Source: CAD feature listing. Evaluate the final solid. Frame: model axes, mm. A direction names the side the tool comes from. Give positions to 0.01 mm unless a question says otherwise; leave off trailing zeros. Order: outer loops, then holes, each group sorted by start corner. A loop starts at its lowest first (then second) coordinate and runs counter-clockwise, first axis right, second up. Notation, with made-up numbers: (13, 5.5) - (51, 5.5) arc R8 ccw to (51, 19.5) - close; hole circle Ø8 at (6, 35). An arc over 180 degrees is marked (long way). Use CSV: the item, a comma, the result in double quotes.
```python
from build123d import *

# Parameters (mm, degrees)
SKETCH1_R           = 1.5
BOSS_EXTRUDE1_DEPTH = 1.75
BOSS_EXTRUDE2_DEPTH = 3
BOSS_EXTRUDE3_DEPTH = 0.5
CUT_EXTRUDE1_REACH  = 5.5
SKETCH4_R           = 0.311736168


with BuildPart() as part:
    # Sketch1 → Boss-Extrude1 (new body)
    with BuildSketch(Plane(origin=(0, 0, 0), x_dir=(1, 0, 0), z_dir=(0, 1, 0))):
        with BuildLine():
            Line((16, -18), (-16, -18))
            ThreePointArc((-16, -18), (-17.414213562, -17.414213562), (-18, -16))
            Line((-18, -16), (-18, 16))
            ThreePointArc((-18, 16), (-17.414213562, 17.414213562), (-16, 18))
            Line((-16, 18), (16, 18))
            ThreePointArc((16, 18), (17.414213562, 17.414213562), (18, 16))
            Line((18, 16), (18, -16))
            ThreePointArc((18, -16), (17.414213562, -17.414213562), (16, -18))
        make_face()
        with Locations((15.25, 15.25)):
            Circle(SKETCH1_R, mode=Mode.SUBTRACT)
        with Locations((-15.25, 15.25)):
            Circle(SKETCH1_R, mode=Mode.SUBTRACT)
        with Locations((15.25, -15.25)):
            Circle(SKETCH1_R, mode=Mode.SUBTRACT)
        with Locations((-15.25, -15.25)):
            Circle(SKETCH1_R, mode=Mode.SUBTRACT)
    extrude(amount=BOSS_EXTRUDE1_DEPTH)

    # Sketch2 → Boss-Extrude2 (add)
    with BuildSketch(Plane.XY.offset(18)):
        with BuildLine():
            Line((4.625773415, 1.75), (8.625773415, 1.75))
            Line((8.625773415, 1.75), (8.625773415, 3.25))
            ThreePointArc((8.625773415, 3.25), (8.596484093, 3.320710678), (8.525773415, 3.35))
            Line((8.525773415, 3.35), (8.325773415, 3.35))
            ThreePointArc((8.325773415, 3.35), (8.255062737, 3.379289322), (8.225773415, 3.45))
            Line((8.225773415, 3.45), (8.225773415, 3.65))
            ThreePointArc((8.225773415, 3.65), (8.196484093, 3.720710678), (8.125773415, 3.75))
            Line((8.125773415, 3.75), (5.125773415, 3.75))
            ThreePointArc((5.125773415, 3.75), (5.055062737, 3.720710678), (5.025773415, 3.65))
            Line((5.025773415, 3.65), (5.025773415, 3.45))
            ThreePointArc((5.025773415, 3.45), (4.996484093, 3.379289322), (4.925773415, 3.35))
            Line((4.925773415, 3.35), (4.725773415, 3.35))
            ThreePointArc((4.725773415, 3.35), (4.655062737, 3.320710678), (4.625773415, 3.25))
            Line((4.625773415, 3.25), (4.625773415, 1.75))
        make_face()
        with BuildLine():
            Line((5.125773415, 3.66), (8.125773415, 3.66))
            ThreePointArc((8.125773415, 3.66), (8.132844483, 3.657071068), (8.135773415, 3.65))
            Line((8.135773415, 3.65), (8.135773415, 3.45))
            ThreePointArc((8.135773415, 3.45), (8.191423127, 3.315649712), (8.325773415, 3.26))
            Line((8.325773415, 3.26), (8.525773415, 3.26))
            ThreePointArc((8.525773415, 3.26), (8.532844483, 3.257071068), (8.535773415, 3.25))
            Line((8.535773415, 3.25), (8.535773415, 1.84))
            Line((8.535773415, 1.84), (4.715773415, 1.84))
            Line((4.715773415, 1.84), (4.715773415, 3.25))
            ThreePointArc((4.715773415, 3.25), (4.718702348, 3.257071068), (4.725773415, 3.26))
            Line((4.725773415, 3.26), (4.925773415, 3.26))
            ThreePointArc((4.925773415, 3.26), (5.060123704, 3.315649712), (5.115773415, 3.45))
            Line((5.115773415, 3.45), (5.115773415, 3.65))
            ThreePointArc((5.115773415, 3.65), (5.118702348, 3.657071068), (5.125773415, 3.66))
        make_face(mode=Mode.SUBTRACT)
    extrude(amount=-BOSS_EXTRUDE2_DEPTH)

    # Sketch3 → Boss-Extrude3 (add)
    with BuildSketch(Plane(origin=(0, 0, 15), x_dir=(-1, 0, 0), z_dir=(0, 0, -1))):
        with BuildLine():
            Line((-4.625773415, 1.75), (-4.625773415, 3.25))
            ThreePointArc((-4.625773415, 3.25), (-4.655062737, 3.320710678), (-4.725773415, 3.35))
            Line((-4.725773415, 3.35), (-4.925773415, 3.35))
            ThreePointArc((-4.925773415, 3.35), (-4.996484093, 3.379289322), (-5.025773415, 3.45))
            Line((-5.025773415, 3.45), (-5.025773415, 3.65))
            ThreePointArc((-5.025773415, 3.65), (-5.055062737, 3.720710678), (-5.125773415, 3.75))
            Line((-5.125773415, 3.75), (-8.125773415, 3.75))
            ThreePointArc((-8.125773415, 3.75), (-8.196484093, 3.720710678), (-8.225773415, 3.65))
            Line((-8.225773415, 3.65), (-8.225773415, 3.45))
            ThreePointArc((-8.225773415, 3.45), (-8.255062737, 3.379289322), (-8.325773415, 3.35))
            Line((-8.325773415, 3.35), (-8.525773415, 3.35))
            ThreePointArc((-8.525773415, 3.35), (-8.596484093, 3.320710678), (-8.625773415, 3.25))
            Line((-8.625773415, 3.25), (-8.625773415, 1.75))
            Line((-8.625773415, 1.75), (-4.625773415, 1.75))
        make_face()
    extrude(amount=BOSS_EXTRUDE3_DEPTH)

    # Sketch4 → Cut-Extrude1 (cut, up to next)
    with BuildSketch(Plane(origin=(0, 0, 14.5), x_dir=(-1, 0, 0), z_dir=(0, 0, -1)), mode=Mode.PRIVATE) as cut_extrude1_sk1:
        with Locations((-5.676091673, 2.531528256)):
            Circle(SKETCH4_R)
    cut_extrude1_tool1 = extrude(cut_extrude1_sk1.sketch, amount=-CUT_EXTRUDE1_REACH, mode=Mode.PRIVATE) & part.part
    add(cut_extrude1_tool1.solids().sort_by_distance((5.676092, 2.531528, 14.5))[0], mode=Mode.SUBTRACT)
    # Sketch4 → Cut-Extrude1 (cut, up to next)
    with BuildSketch(Plane(origin=(0, 0, 14.5), x_dir=(-1, 0, 0), z_dir=(0, 0, -1)), mode=Mode.PRIVATE) as cut_extrude1_sk2:
        with Locations((-7.641197668, 2.531528256)):
            Circle(SKETCH4_R)
    cut_extrude1_tool2 = extrude(cut_extrude1_sk2.sketch, amount=-CUT_EXTRUDE1_REACH, mode=Mode.PRIVATE) & part.part
    add(cut_extrude1_tool2.solids().sort_by_distance((7.641198, 2.531528, 14.5))[0], mode=Mode.SUBTRACT)
    # Sketch4 → Cut-Extrude1 (cut, up to next)
    with BuildSketch(Plane(origin=(0, 0, 14.5), x_dir=(-1, 0, 0), z_dir=(0, 0, -1)), mode=Mode.PRIVATE) as cut_extrude1_sk3:
        with Locations((-6.649897908, 2.531528256)):
            Circle(SKETCH4_R)
    cut_extrude1_tool3 = extrude(cut_extrude1_sk3.sketch, amount=-CUT_EXTRUDE1_REACH, mode=Mode.PRIVATE) & part.part
    add(cut_extrude1_tool3.solids().sort_by_distance((6.649898, 2.531528, 14.5))[0], mode=Mode.SUBTRACT)


solid = part.part
```
Item 1: First-contact query: pin 1 (0.5 mm diameter, centred on x = 7, y = 3, fed in from +Z); pin 2 (1.2 mm diameter, centred on y = 2.5, z = 16.5, fed in from -X); pin 3 (1 mm diameter, centred on x = 11.5, z = 13, fed in from +Y). Flat tips, straight axial feed; report the tip coordinate or a pass-through.
Filled in:
pin 1,"stops at z = 15"
pin 2,"stops at x = 4.63"
pin 3,"stops at y = 1.75"
Item 2: Set-up query: faces 4 (the flat face through (7, 1.84, 17)), 5 (the cylindrical face through (-17.43, 0.86, -17.4)). Return all of +Z, -Z, +X, -X, +Y, -Y with unobstructed straight access to the full face (end or side cutting, diameter ignored); none if empty.
Filled in:
face 4,"+Z"
face 5,"-Z, -X, +Y, -Y"
Item 3: Material intervals for line 1 (X direction, y = 0.9, z = -15.25); line 2 (X direction, y = 0.5, z = 16), sorted ascending. Write a range as from..to.
Filled in:
line 1,"x = -18..-16.75, -13.75..13.75, 16.75..18"
line 2,"x = -18..-16.55, -13.95..13.95, 16.55..18"
Item 4: Mould query, pull axis X, two halves, no side actions, for faces 1 (the cylindrical face through (13.75, 0.86, 15.18)), 2 (the cylindrical face through (-17.4, 0.86, 17.43)), 3 (the flat face through (0, 1, -18)). Classes: released by +X, released by -X, zero draft, split by the parting line, or undercut.
Filled in:
face 1,"undercut"
face 2,"released by -X"
face 3,"zero draft"
Item 5: Section C-C on z = 10.5. Return the cut outline in (x, y), then the cut area to 3 significant figures.
Filled in:
outline,"(-18, 0) - (18, 0) - (18, 1.75) - (-18, 1.75) - close"
area,"63.0 mm2"
Item 6: Section A-A on y = 1. Return the cut outline in (x, z), then the cut area to 3 significant figures.
Filled in:
outline,"(-18, -16) arc R2 ccw to (-16, -18) - (16, -18) arc R2 ccw to (18, -16) - (18, 16) arc R2 ccw to (16, 18) - (-16, 18) arc R2 ccw to (-18, 16) - close; hole circle Ø3 at (-15.25, -15.25); hole circle Ø3 at (-15.25, 15.25); hole circle Ø3 at (15.25, -15.25); hole circle Ø3 at (15.25, 15.25)"
area,"1,260 mm2"
Item 7: Section B-B on x = -15.25. Return the cut outline in (y, z), then the cut area to 3 significant figures.
Filled in:
outline,"(0, -18) - (1.75, -18) - (1.75, -16.75) - (0, -16.75) - close; (0, -13.75) - (1.75, -13.75) - (1.75, 13.75) - (0, 13.75) - close; (0, 16.75) - (1.75, 16.75) - (1.75, 18) - (0, 18) - close"
area,"52.5 mm2"
